Check sheet for the modelled part. Datum: model origin and axes. Units: mm. Face numbers are marked on the shaded views. A direction names the side the tool comes from. Give positions to 0.01 mm unless a question says otherwise; leave off trailing zeros. Order: outer loops, then holes, each group sorted by start corner. A loop starts at its lowest first (then second) coordinate and runs counter-clockwise, first axis right, second up. Notation, with made-up numbers: (68, 9) - (97, 9) arc R19 cw to (97, 18) - close; hole circle Ø9 at (85.25, -6.75). An arc over 180 degrees is marked (long way). Answer in a Markdown table with one row per item.
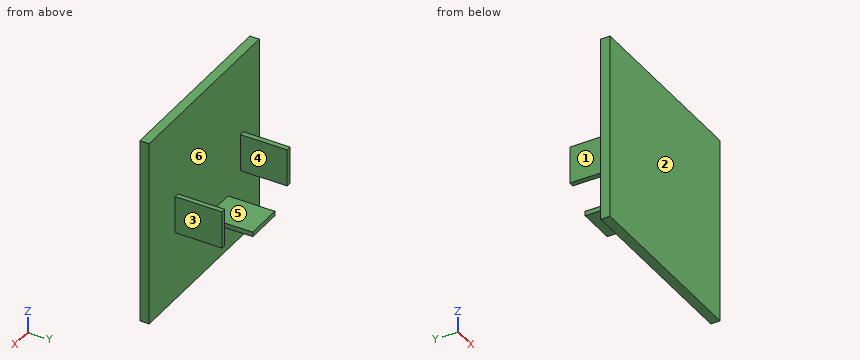
from build123d import *

# Parameters (mm, degrees)
SKETCH1_W           = 50.8
SKETCH1_H           = 2.54
BOSS_EXTRUDE1_DEPTH = 50.8
SKETCH2_W           = 10.16
SKETCH2_H           = 1.27
SKETCH2_W_2         = 1.27
SKETCH2_H_2         = 10.16
SKETCH2_W_3         = 1.379502468
BOSS_EXTRUDE2_DEPTH = 12.7


with BuildPart() as part:
    # Sketch1 → Boss-Extrude1 (new body)
    with BuildSketch(Plane.XY):
        with Locations((-118.555926356, -26.291516762)):
            Rectangle(SKETCH1_W, SKETCH1_H)
    extrude(amount=BOSS_EXTRUDE1_DEPTH)

    # Sketch2 → Boss-Extrude2 (add)
    with BuildSketch(Plane(origin=(0, -25.021516762, 0), x_dir=(1, 0, 0), z_dir=(0, 1, 0))):
        with Locations((-124.433948154, -14.360513522)):
            Rectangle(SKETCH2_W, SKETCH2_H)
        with Locations((-105.788523286, -23.868729288)):
            Rectangle(SKETCH2_W_2, SKETCH2_H_2)
        with Locations((-135.937615572, -23.868729288)):
            Rectangle(SKETCH2_W_3, SKETCH2_H_2)
    extrude(amount=BOSS_EXTRUDE2_DEPTH)


solid = part.part
(1) Cross-section at C-C, the plane z = 10. Record the cut outline in (x, y).
Geometry says:
| item | result |
|---|---|
| outline | (-143.96, -27.56) - (-93.16, -27.56) - (-93.16, -25.02) - (-143.96, -25.02) - close |
(2) Cross-section at A-A, the plane y = -15. Record the cut outline in (x, z), then the cut area to 3 significant figures.
Geometry says:
| item | result |
|---|---|
| outline | (-136.63, 18.79) - (-135.25, 18.79) - (-135.25, 28.95) - (-136.63, 28.95) - close; (-129.51, 13.73) - (-119.35, 13.73) - (-119.35, 15) - (-129.51, 15) - close; (-106.42, 18.79) - (-105.15, 18.79) - (-105.15, 28.95) - (-106.42, 28.95) - close |
| area | 39.8 mm² |
(3) Thickness scan on L1, parallel to Y at x = -100.5, z = 33; L2, parallel to X at y = -15, z = 27.5; L3, parallel to Z at x = -126, y = -17.5. Record the ranges inside material, lowest first.
Geometry says:
| item | result |
|---|---|
| L1 | -27.56 to -25.02 |
| L2 | -136.63 to -135.25, -106.42 to -105.15 |
| L3 | 13.73 to 15 |
(4) Cross-section at B-B, the plane x = -126.5. Record the cut outline in (y, z).
Geometry says:
| item | result |
|---|---|
| outline | (-27.56, 0) - (-25.02, 0) - (-25.02, 13.73) - (-12.32, 13.73) - (-12.32, 15) - (-25.02, 15) - (-25.02, 50.8) - (-27.56, 50.8) - close |
(5) Access from +Z, -Z, +X, -X, +Y, -Y to the whole of each face (thin tool, end or side, straight path). Record for the marked faces 1, 2, 3 and 4.
Geometry says:
| item | result |
|---|---|
| face 1 | +Z, -Z, -X, +Y |
| face 2 | +Z, -Z, +X, -X, -Y |
| face 3 | +Z, -Z, +X, +Y |
| face 4 | +Z, -Z, +Y |
(6) Gauge pin test, flat ends, axial feed: P1, Ø1.5, axis at x = -107.5, y = -14.5, coming from the -Z side; P2, Ø6, axis at x = -121.5, z = 33.5, coming from the +Y side; P3, Ø5, axis at x = -123, y = -19, coming from the -Z side; P4, Ø3, axis at y = -16, z = 22.5, coming from the -X side. Record the tip position at first contact, or that the pin passes through.
Geometry says:
| item | result |
|---|---|
| P1 | through |
| P2 | y = -25.02 |
| P3 | z = 13.73 |
| P4 | x = -136.63 |
(7) Mould release check, pull along Z, two halves, no side actions. Record for the marked faces 5 and 6: pulls with the +Z half, pulls with the -Z half, needs draft (parallel to the pull), parting line crosses it, or undercut.
Geometry says:
| item | result |
|---|---|
| face 5 | pulls with the +Z half |
| face 6 | needs draft |
(8) Cross-section at D-D, the plane x = -109. Record the cut outline in (y, z), then the cut area to 3 significant figures.
Geometry says:
| item | result |
|---|---|
| outline | (-27.56, 0) - (-25.02, 0) - (-25.02, 50.8) - (-27.56, 50.8) - close |
| area | 129 mm² |
